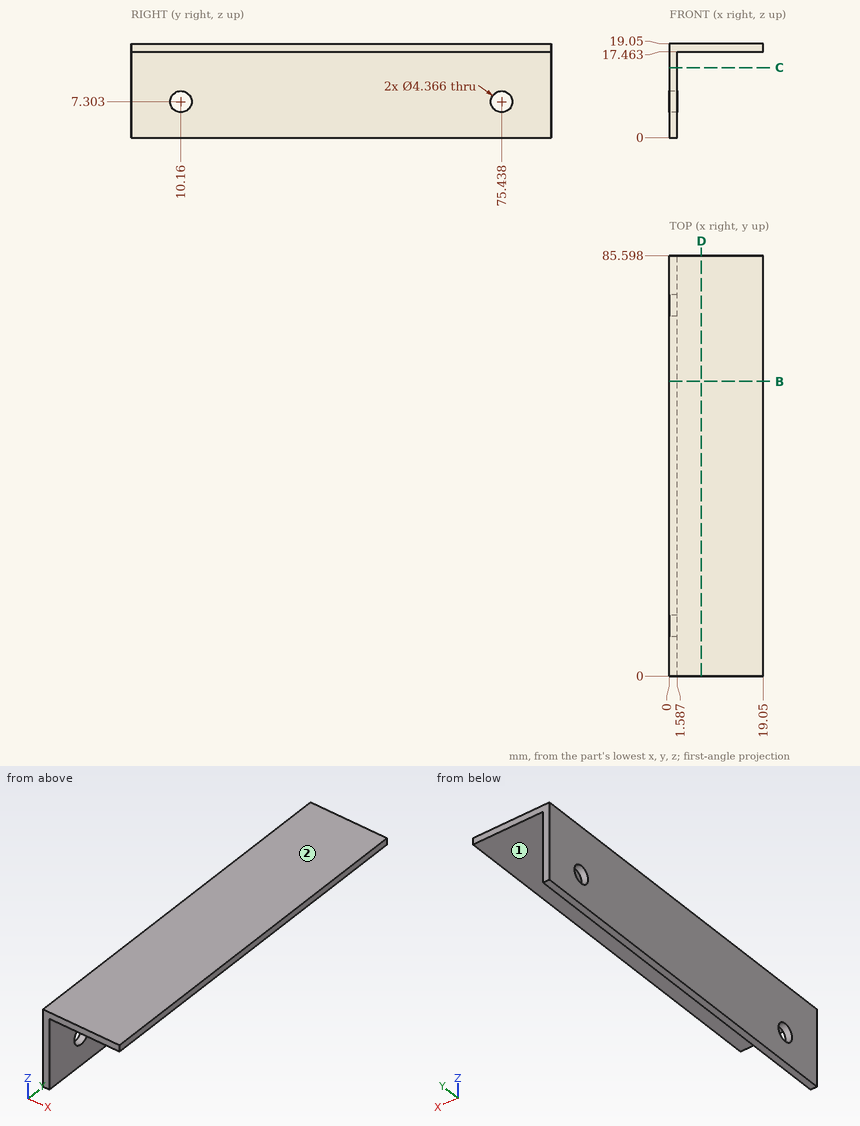
Check sheet for the drawn part. Datum: minimum x, y, z corner. Units: mm. A direction names the side the tool comes from. Give positions to 0.01 mm unless a question says otherwise; leave off trailing zeros. Loops run counter-clockwise (first coordinate to the right, second up) from the corner with the lowest first, then second, coordinate; pieces in that order, holes last. Notation, with made-up numbers: (18.25, -26.75) - (31.25, -26.75) arc R11 cw to (31.25, -20.75) - close; hole circle Ø11 at (-17, 70.25). An arc over 180 degrees is marked (long way). Write each question's results on one line, items separated by ' | '.
1) Sectioned sample at D-D on x = 6.5. Record the boundary of the cut face in (y, z), plus the area to 3 significant figures.
Solution:
outline: (0, 17.46) - (85.6, 17.46) - (85.6, 19.05) - (0, 19.05) - close | area: 136 mm2
2) Tool access check on the marked faces 1 and 2. Record the directions out of +Z, -Z, +X, -X, +Y, -Y that give a thin tool (end or side, any length) a straight path to the whole face; none if there is none.
Solution:
face 1: -Z, +X, +Y, -Y | face 2: +Z, +X, -X, +Y, -Y
3) Depth check by flat-ended pin: P1, Ø5, axis at x = 7.5, z = 16, coming from the +Y side; P2, Ø7, axis at y = 10.16, z = 7.3, coming from the +X side; P3, Ø5, axis at x = 10, y = 55.5, coming from the -Z side. Enter the tip coordinate at first touch or a pass-through.
Solution:
P1: y = 85.6 | P2: x = 1.59 | P3: z = 17.46
4) Sectioned sample at B-B on y = 60. Record the boundary of the cut face in (x, z).
Solution:
outline: (0, 0) - (1.59, 0) - (1.59, 17.46) - (19.05, 17.46) - (19.05, 19.05) - (0, 19.05) - close
5) Sectioned sample at C-C on z = 14.25. Record the boundary of the cut face in (x, y), plus the area to 3 significant figures.
Solution:
outline: (0, 0) - (1.59, 0) - (1.59, 85.6) - (0, 85.6) - close | area: 136 mm2
6) Material ranges on L1, parallel to X at y = 67, z = 16.75; L2, parallel to Z at x = 12.5, y = 79.5, recorded low to high. Write a range as from..to.
Solution:
L1: 0..1.59 | L2: 17.46..19.05
